```python
from build123d import *

# Parameters (mm, degrees)
SKETCH1_W           = 50
SKETCH1_H           = 30
SKETCH1_R           = 1.5
BOSS_EXTRUDE1_DEPTH = 4
SKETCH2_W           = 21
SKETCH2_H           = 30
CUT_EXTRUDE1_DEPTH  = 1.5
SKETCH3_R           = 1.75
CUT_EXTRUDE2_DEPTH  = 5


with BuildPart() as part:
    # Sketch1 → Boss-Extrude1 (new body)
    with BuildSketch(Plane.XY):
        with Locations((25, 15)):
            Rectangle(SKETCH1_W, SKETCH1_H)
        with Locations((6, 25)):
            Circle(SKETCH1_R, mode=Mode.SUBTRACT)
        with Locations((44, 5)):
            Circle(SKETCH1_R, mode=Mode.SUBTRACT)
    extrude(amount=BOSS_EXTRUDE1_DEPTH)

    # Sketch2 → Cut-Extrude1 (cut)
    with BuildSketch(Plane.XY.offset(4)):
        with Locations((25, 15)):
            Rectangle(SKETCH2_W, SKETCH2_H)
    extrude(amount=-CUT_EXTRUDE1_DEPTH, mode=Mode.SUBTRACT)

    # Sketch3 → Cut-Extrude2 (cut)
    with BuildSketch(Plane.XY.offset(2.5)):
        with Locations((25, 25)):
            Circle(SKETCH3_R)
        with Locations((25, 5)):
            Circle(SKETCH3_R)
    extrude(amount=-CUT_EXTRUDE2_DEPTH, mode=Mode.SUBTRACT)


solid = part.part
```
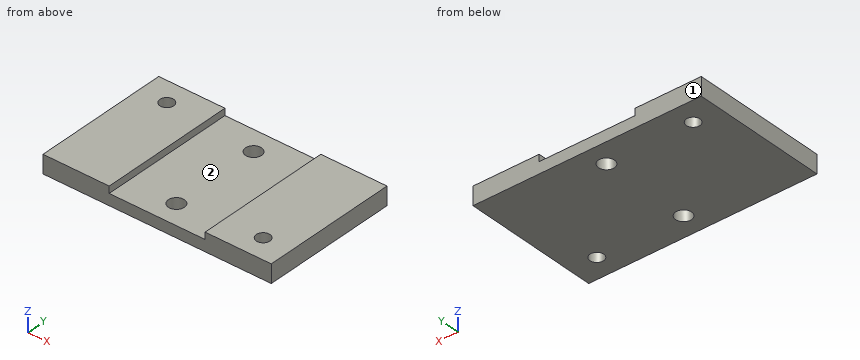
The listing builds one solid part. Answer for the finished solid, in the listing's coordinates (mm). Face numbers are marked on the shaded views. A direction names the side the tool comes from. Give positions to 0.01 mm unless a question says otherwise; leave off trailing zeros. Write each loop counter-clockwise with the first axis right and the second up, starting at its lowest first coordinate (ties: lowest second). Pieces come first, ordered by that corner, then holes. Notation, with made-up numbers: M -26.5,58.5 L -22.5,58.5 A22 cw -22.5,76.5 Z; hole C 78.5,7.25 d9. An arc over 180 degrees is marked long. Write each question's results on one line, items separated by ' | '.
Q1. Section B-B, the plane x = 44 is taken. Write down the section's boundary in (y, z).
Output values:
outline: M 0,0 L 3.5,0 L 3.5,4 L 0,4 Z; M 6.5,0 L 30,0 L 30,4 L 6.5,4 Z
Q2. Flat-ended cylindrical pins translate along their axes: P1, Ø2, axis at y = 14, z = 2.5, coming from the -X side; P2, Ø12, axis at x = 29, y = 11, coming from the +Z side. Find the tip coordinate at first contact, or state that the pin passes through.
Output values:
P1: x = 0 | P2: z = 2.5
Q3. Section D-D, the plane x = 26 is taken. Write down the section's boundary in (y, z).
Output values:
outline: M 0,0 L 3.56,0 L 3.56,2.5 L 0,2.5 Z; M 6.44,0 L 23.56,0 L 23.56,2.5 L 6.44,2.5 Z; M 26.44,0 L 30,0 L 30,2.5 L 26.44,2.5 Z
Q4. Section C-C, the plane z = 1.65 is taken. Write down the section's boundary in (x, y).
Output values:
outline: M 0,0 L 50,0 L 50,30 L 0,30 Z; hole C 6,25 d3; hole C 25,5 d3.5; hole C 25,25 d3.5; hole C 44,5 d3
Q5. Consider L1, parallel to Y at x = 25, z = 1.8; L2, parallel to X at y = 22.25, z = 2.6; L3, parallel to Y at x = 26.5, z = 0.75. Determine where each line is inside the solid, lowest interval first. Write a range as from..to.
Output values:
L1: 0..3.25, 6.75..23.25, 26.75..30 | L2: 0..14.5, 35.5..50 | L3: 0..4.1, 5.9..24.1, 25.9..30
Q6. A tool of negligible diameter and unlimited length cuts with its end or side. For the marked faces 1 and 2, from which of +Z, -Z, +X, -X, +Y, -Y can it reach the whole face along a straight path? Write none if from no direction.
Output values:
face 1: +Z, -Z, +X, -X, +Y | face 2: +Z, +Y, -Y
Q7. Section A-A, the plane y = 5 is taken. Write down the section's boundary in (x, z), then the cut area to 3 significant figures.
Output values:
outline: M 0,0 L 23.25,0 L 23.25,2.5 L 14.5,2.5 L 14.5,4 L 0,4 Z; M 26.75,0 L 42.5,0 L 42.5,4 L 35.5,4 L 35.5,2.5 L 26.75,2.5 Z; M 45.5,0 L 50,0 L 50,4 L 45.5,4 Z | area: 148 mm2
